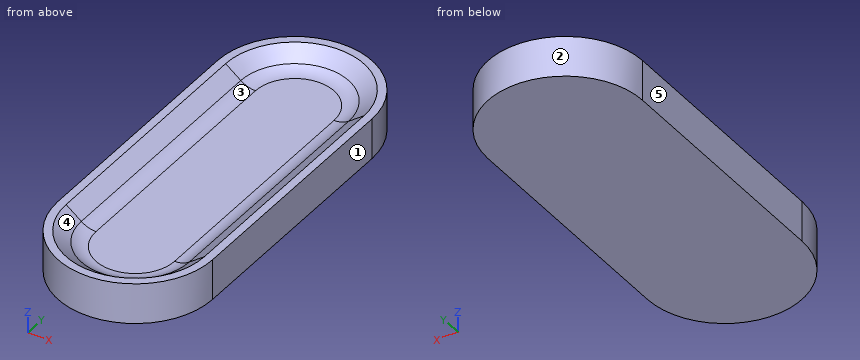
```python
from build123d import *

# Parameters (mm, degrees)
Y_KSEKLIK_EKSTR_ZYON1_DEPTH = 5
KES_EKSTR_ZYON1_DEPTH       = 2
PAH1_SIZE                   = 4
PAH1_SIZE_2                 = 3
RADYUS1_R                   = 3


with BuildPart() as part:
    # Çizim1 → Yükseklik-Ekstrüzyon1 (new body)
    with BuildSketch(Plane.XY):
        with BuildLine():
            Line((-9.5, -15), (-9.5, 15))
            ThreePointArc((-9.5, 15), (0, 24.5), (9.5, 15))
            Line((9.5, 15), (9.5, -15))
            ThreePointArc((9.5, -15), (0, -24.5), (-9.5, -15))
        make_face()
    extrude(amount=Y_KSEKLIK_EKSTR_ZYON1_DEPTH)

    # Çizim2 → Kes-Ekstrüzyon1 (cut)
    with BuildSketch(Plane.XY.offset(5)):
        with BuildLine():
            Line((-4.5, 15), (-4.5, -15))
            ThreePointArc((-4.5, -15), (0, -19.5), (4.5, -15))
            Line((4.5, -15), (4.5, 15))
            ThreePointArc((4.5, 15), (0, 19.5), (-4.5, 15))
        make_face()
    extrude(amount=-KES_EKSTR_ZYON1_DEPTH, mode=Mode.SUBTRACT)

    # Pah1
    # the kernel refuses this chamfer: 4, 3 mm, written as the material it takes off along each edge
    with BuildSketch(Plane(origin=(0, -15, 5), x_dir=(-1, 0, 0), z_dir=(0, 1, 0))) as pah1_piece_1_section:
        Polygon((4.5 + PAH1_SIZE, 0), (4.5, -PAH1_SIZE_2), (4.5, 0), align=None)
    pah1_piece_1 = revolve(axis=Axis((0, -15, 5), (0, 0, 1)), revolution_arc=180, mode=Mode.PRIVATE)
    pah1_piece_1 = split(pah1_piece_1, bisect_by=Plane(origin=(0, -22.201904041, 3), z_dir=(0, 0, 1)), keep=Keep.TOP, mode=Mode.PRIVATE)
    add(pah1_piece_1, mode=Mode.SUBTRACT)
    with BuildSketch(Plane(origin=(4.5, -15, 5), x_dir=(0.9997296931968459, 0, 0.023249527748763873), z_dir=(0, 1, 0))) as pah1_piece_2_section:
        Polygon((PAH1_SIZE * 0.999729693197, PAH1_SIZE * 0.0232495277488), (-PAH1_SIZE_2 * 0.0232495277488, PAH1_SIZE_2 * 0.999729693197), (0, 0), align=None)
    pah1_piece_2 = extrude(amount=30, mode=Mode.PRIVATE)
    pah1_piece_2 = split(pah1_piece_2, bisect_by=Plane(origin=(5.968375105, 0, 3), z_dir=(0, 0, 1)), keep=Keep.TOP, mode=Mode.PRIVATE)
    add(pah1_piece_2, mode=Mode.SUBTRACT)
    with BuildSketch(Plane(origin=(-4.5, 15, 5), x_dir=(-0.9997296931968459, 0, 0.023249527748763883), z_dir=(0, -1, 0))) as pah1_piece_3_section:
        Polygon((PAH1_SIZE * 0.999729693197, PAH1_SIZE * 0.0232495277488), (-PAH1_SIZE_2 * 0.0232495277488, PAH1_SIZE_2 * 0.999729693197), (0, 0), align=None)
    pah1_piece_3 = extrude(amount=30, mode=Mode.PRIVATE)
    pah1_piece_3 = split(pah1_piece_3, bisect_by=Plane(origin=(-5.968375105, 0, 3), z_dir=(0, 0, 1)), keep=Keep.TOP, mode=Mode.PRIVATE)
    add(pah1_piece_3, mode=Mode.SUBTRACT)
    with BuildSketch(Plane(origin=(0, 15, 5), x_dir=(1, 0, 0), z_dir=(0, -1, 0))) as pah1_piece_4_section:
        Polygon((4.5 + PAH1_SIZE, 0), (4.5, -PAH1_SIZE_2), (4.5, 0), align=None)
    pah1_piece_4 = revolve(axis=Axis((0, 15, 5), (0, 0, 1)), revolution_arc=180, mode=Mode.PRIVATE)
    pah1_piece_4 = split(pah1_piece_4, bisect_by=Plane(origin=(0, 22.201904042, 3), z_dir=(0, 0, 1)), keep=Keep.TOP, mode=Mode.PRIVATE)
    add(pah1_piece_4, mode=Mode.SUBTRACT)

    # Radyus1
    radyus1_edges = [part.edges().sort_by_distance(p)[0] for p in [
        (0, -20.833333333, 3),
        (5.833333333, 0, 3),
        (-5.833333333, 0, 3),
        (0, 20.833333333, 3),
    ]]
    fillet(radyus1_edges, radius=RADYUS1_R)


solid = part.part
```
Build history of the part. All positions in model axes, mm. Face numbers are marked on the shaded views. A direction names the side the tool comes from. Round coordinates to 2 decimals unless told otherwise and drop trailing zeros. Write each loop counter-clockwise with the first axis right and the second up, starting at its lowest first coordinate (ties: lowest second). Pieces come first, ordered by that corner, then holes. Notation, with made-up numbers: (3.5, 36.25) -> (54.5, 36.25) arc R16 ccw to (54.5, 52.25) -> close; hole circle Ø7 at (-33, 42.5). An arc over 180 degrees is marked (long way). Put each result on its own line as item: value.
Item 1: Flat gauge pins, fed straight in: P1, Ø5, axis at x = -2, y = -9.5, coming from the +Z side; P2, Ø2, axis at x = -2, z = 2, coming from the +Y side; P3, Ø2, axis at x = -3, z = 1.5, coming from the +Y side. Where does each tip first touch, or does it go through?
Here are the results:
P1: stops at z = 3
P2: stops at y = 24.45
P3: stops at y = 24.29
Item 2: Slice it at C-C, the plane z = 2. Give the cut face in (x, y), plus the area to 3 significant figures.
Here are the results:
outline: (-9.5, -15) arc R9.5 ccw to (9.5, -15) -> (9.5, 15) arc R9.5 ccw to (-9.5, 15) -> close
area: 854 mm^2
Item 3: Two-plate mould, pull along Y, no slides. Class the marked faces 1, 2 and 3: pulls with the +Y half, pulls with the -Y half, needs draft (parallel to the pull), parting line crosses it, or undercut.
Here are the results:
face 1: needs draft
face 2: pulls with the +Y half
face 3: undercut
Item 4: Slice it at A-A, the plane y = 9. Give the cut face in (x, z).
Here are the results:
outline: (-9.5, 0) -> (9.5, 0) -> (9.5, 5) -> (8.5, 5) -> (6.63, 3.6) arc R3 cw to (4.83, 3) -> (-4.83, 3) arc R3 cw to (-6.63, 3.6) -> (-8.5, 5) -> (-9.5, 5) -> close
Item 5: Tool access for the marked faces 4 and 5: list every direction of +Z, -Z, +X, -X, +Y, -Y with a clear straight run to the whole face (end or side of a thin tool).
Here are the results:
face 4: +Z
face 5: +Z, -Z, -X, +Y, -Y
Item 6: Wall check: probe 1 along Z at (x, y) = (2.25, 8.5); probe 2 along Y at (x, z) = (0, 4.2); probe 3 along Y at (x, z) = (5.25, 4.3). Give the ranges that are in metal, low to high. Write a range as from..to.
Here are the results:
probe 1: z = 0..3
probe 2: y = -24.5..-22.43, 22.43..24.5
probe 3: y = -22.92..-20.45, 20.45..22.92
Item 7: Slice it at B-B, the plane x = 0. Give the cut face in (y, z).
Here are the results:
outline: (-24.5, 0) -> (24.5, 0) -> (24.5, 5) -> (23.5, 5) -> (21.63, 3.6) arc R3 cw to (19.83, 3) -> (-19.83, 3) arc R3 cw to (-21.63, 3.6) -> (-23.5, 5) -> (-24.5, 5) -> close
